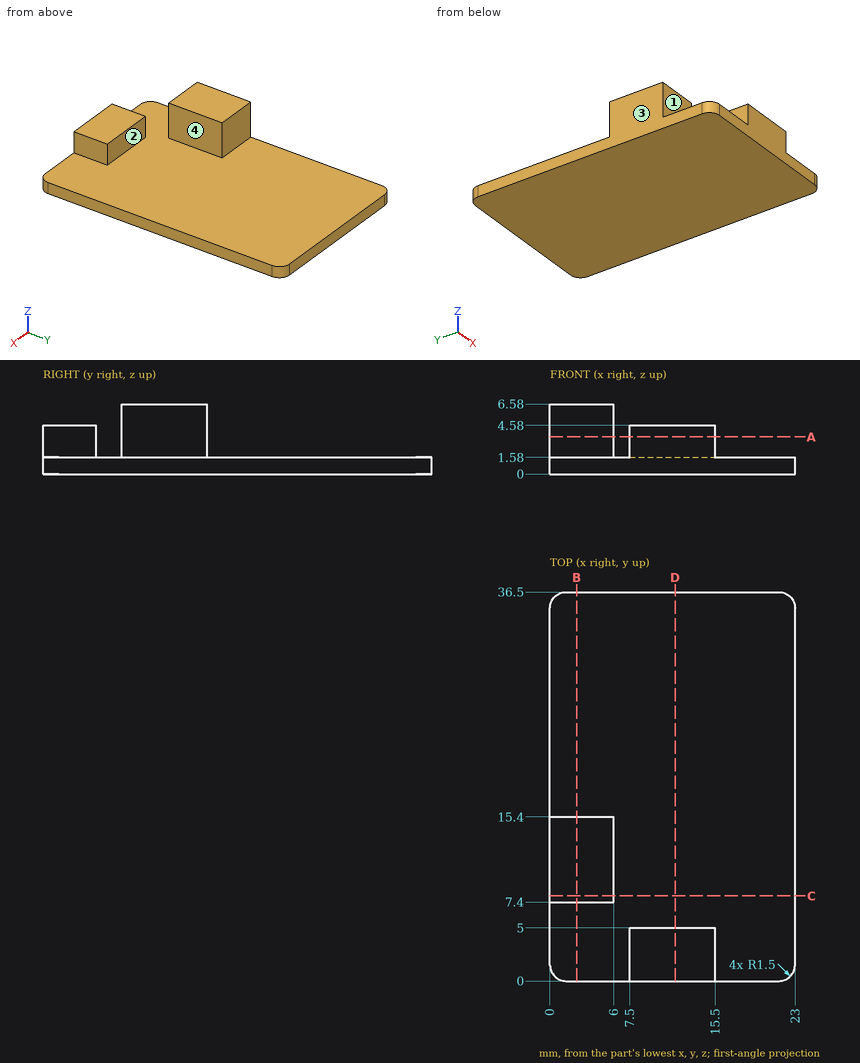
Design review of the part shown in the three views and the two pictorial views. Dimensions are in mm from the part's minimum x, y and z. A direction names the side the tool comes from. Round coordinates to 2 decimals unless told otherwise and drop trailing zeros. Write each loop counter-clockwise with the first axis right and the second up, starting at its lowest first coordinate (ties: lowest second). Pieces come first, ordered by that corner, then holes. Notation, with made-up numbers: (82, 19) -> (133, 19) arc R26 ccw to (133, 50) -> close; hole circle Ø8 at (-7.5, 42). An arc over 180 degrees is marked (long way). One line per question, with ' | ' between items. Start each with the question number.
1) Add section A-A (z = 3.5). Write out the cut boundary in (x, y).
2) Machinability: for the marked faces 1, 2, 3 and 4, which of the approach directions +Z, -Z, +X, -X, +Y, -Y give a long, thin tool a straight path to every point of the face, cutting with its end or side? Answer none if there is none.
3) Wall thickness on line 1 along X through (y, z) = (10, 4.25); line 2 along Z through (x, y) = (8, 35); line 3 along Z through (x, y) = (11.25, 2): over which ranges is each line inside the solid? List them lowest first.
4) Add section C-C (y = 8). Write out the cut boundary in (x, z), and give its area (3 significant figures).
5) For pin 1 Ø1.5 at (x, y) = (12.5, 3.5) entering from +Z; pin 2 Ø1.5 at (x, z) = (4, 5) entering from -Y; pin 3 Ø2.5 at (x, z) = (1.5, 5) entering from +Y, all flat-tipped, find the tip position at first contact; note any pin that passes through.
6) Add section B-B (x = 2.5). Write out the cut boundary in (y, z), and give its area (3 significant figures).
7) Add section D-D (x = 11.75). Write out the cut boundary in (y, z), and give its area (3 significant figures).
Reported:
1) outline: (0, 7.4) -> (6, 7.4) -> (6, 15.4) -> (0, 15.4) -> close; (7.5, 0) -> (15.5, 0) -> (15.5, 5) -> (7.5, 5) -> close
2) face 1: +Z, +X, -X, -Y | face 2: +Z, +X, -X, +Y | face 3: +Z, -Z, -X, +Y, -Y | face 4: +Z, +X, +Y, -Y
3) line 1: x = 0 to 6 | line 2: z = 0 to 1.58 | line 3: z = 0 to 4.58
4) outline: (0, 0) -> (23, 0) -> (23, 1.58) -> (6, 1.58) -> (6, 6.58) -> (0, 6.58) -> close | area: 66.3 mm²
5) pin 1: stops at z = 4.58 | pin 2: stops at y = 7.4 | pin 3: stops at y = 15.4
6) outline: (0, 0) -> (36.5, 0) -> (36.5, 1.58) -> (15.4, 1.58) -> (15.4, 6.58) -> (7.4, 6.58) -> (7.4, 1.58) -> (0, 1.58) -> close | area: 97.7 mm²
7) outline: (0, 0) -> (36.5, 0) -> (36.5, 1.58) -> (5, 1.58) -> (5, 4.58) -> (0, 4.58) -> close | area: 72.7 mm²
